from build123d import *

# Parameters (mm, degrees)
SKETCH1_W                                          = 14.224
SKETCH1_H                                          = 8.636
CBORE_FOR_M2_5_HEX_HEAD_MACHINE_SCREW1_D           = 3.048
CBORE_FOR_M2_5_HEX_HEAD_MACHINE_SCREW1_CBORE_D     = 4.7752
CBORE_FOR_M2_5_HEX_HEAD_MACHINE_SCREW1_CBORE_DEPTH = 3.048
M2_5_CLEARANCE_HOLE1_D                             = 3.048
M2_5_CLEARANCE_HOLE1_DEPTH                         = 2.54
M13_CLEARANCE_HOLE1_D                              = 15.494
M13_CLEARANCE_HOLE1_DEPTH                          = 2.54
CBORE_FOR_M3_5_HEX_HEAD_MACHINE_SCREW1_D           = 3.96748
CBORE_FOR_M3_5_HEX_HEAD_MACHINE_SCREW1_DEPTH       = 7.112
CBORE_FOR_M3_5_HEX_HEAD_MACHINE_SCREW1_CBORE_D     = 7.9375
CBORE_FOR_M3_5_HEX_HEAD_MACHINE_SCREW1_CBORE_DEPTH = 0.508
CBORE_FOR_M3_5_HEX_HEAD_MACHINE_SCREW1_TIP         = 1.145312823
CHAMFER1_SIZE                                      = 0.42926


with BuildPart() as part:
    # Sketch1 → Revolve1 (revolve)
    with BuildSketch(Plane(origin=(0, 0, 0), x_dir=(-1, 0, 0), z_dir=(0, 0, -1)), mode=Mode.PRIVATE) as revolve1_sk:
        with Locations((-7.112, 4.318)):
            Rectangle(SKETCH1_W, SKETCH1_H)
    revolve(revolve1_sk.sketch.rotate(Axis((0, 0, 0), (0, 1, 0)), 270), axis=Axis((0, 0, 0), (0, 1, 0)))

    # CBORE for M2.5 Hex Head Machine Screw1 (through all)
    with Locations(Plane(origin=(0, 8.636, 0), x_dir=(1, 0, 0), z_dir=(0, 1, 0))):
        with Locations((0, -11.176), (0, 11.176)):
            CounterBoreHole(CBORE_FOR_M2_5_HEX_HEAD_MACHINE_SCREW1_D / 2, CBORE_FOR_M2_5_HEX_HEAD_MACHINE_SCREW1_CBORE_D / 2, CBORE_FOR_M2_5_HEX_HEAD_MACHINE_SCREW1_CBORE_DEPTH)

    # M2.5 Clearance Hole1
    with Locations(Plane(origin=(0, 0, 0), x_dir=(-1, 0, 0), z_dir=(0, -1, 0))):
        with Locations((-7.902625387, 7.902625387), (7.902625387, -7.902625387), (-7.902625387, -7.902625387), (7.902625387, 7.902625387)):
            Hole(M2_5_CLEARANCE_HOLE1_D / 2, depth=M2_5_CLEARANCE_HOLE1_DEPTH)

    # M13 Clearance Hole1
    with Locations(Plane(origin=(0, 0, 0), x_dir=(-1, 0, 0), z_dir=(0, -1, 0))):
        with Locations((0, 0)):
            Hole(M13_CLEARANCE_HOLE1_D / 2, depth=M13_CLEARANCE_HOLE1_DEPTH)

    # CBORE for M3.5 Hex Head Machine Screw1
    with Locations(Plane(origin=(-14.224, 5.08, 0), x_dir=(0, 0, -1), z_dir=(-1, 0, 0))):
        with Locations((0, 0)):
            CounterBoreHole(CBORE_FOR_M3_5_HEX_HEAD_MACHINE_SCREW1_D / 2, CBORE_FOR_M3_5_HEX_HEAD_MACHINE_SCREW1_CBORE_D / 2, CBORE_FOR_M3_5_HEX_HEAD_MACHINE_SCREW1_CBORE_DEPTH, depth=CBORE_FOR_M3_5_HEX_HEAD_MACHINE_SCREW1_DEPTH)
            with Locations((0, 0, -(CBORE_FOR_M3_5_HEX_HEAD_MACHINE_SCREW1_DEPTH + CBORE_FOR_M3_5_HEX_HEAD_MACHINE_SCREW1_TIP / 2))):  # 120° drill point
                Cone(0, CBORE_FOR_M3_5_HEX_HEAD_MACHINE_SCREW1_D / 2, CBORE_FOR_M3_5_HEX_HEAD_MACHINE_SCREW1_TIP, mode=Mode.SUBTRACT)

    # Chamfer1
    chamfer1_edges = [part.edges().sort_by_distance(p)[0] for p in [
        (-13.716, 5.08, -1.98374),
    ]]
    chamfer(chamfer1_edges, length=CHAMFER1_SIZE)


solid = part.part
Can you work these out from the model? Positions are in its coordinate system, mm. A direction names the side the tool comes from. Coordinates: 2 decimals unless noted, no trailing zeros. Loops run counter-clockwise (first coordinate to the right, second up) from the corner with the lowest first, then second, coordinate; pieces in that order, holes last. Notation, with made-up numbers: M 66,51 L 115,51 A35 ccw 115,90 Z; hole C 42,-10 d11. An arc over 180 degrees is marked long. Return JSON: item names as keys, results as strings. Group by question number.
Item 1: Imagine slicing it at B-B (x = 0). Please give me the cut outline in (y, z), and give its area (3 significant figures).
Item 2: Imagine slicing it at A-A (z = 10). Please give me the cut outline in (x, y), and give its area (3 significant figures).
Item 3: Thinking about a two-plate mould opening in Z: for faces 1 (the flat face through (0, 8.636, 0)), 2 (the flat face through (-8, 2.54, 8)), which applies, released by +Z, released by -Z, zero draft, split by the parting line, or undercut?
Item 4: Imagine slicing it at C-C (x = -9). Please give me the cut outline in (y, z), and give its area (3 significant figures).
Item 5: I'm going to push flat-ended pins straight in: pin 1 Ø1.5 at (y, z) = (1.5, -1.5) entering from -X; pin 2 Ø1.8 at (x, z) = (7.9, 7.9) entering from -Y; pin 3 Ø4 at (x, z) = (0, 11.176) entering from -Y; pin 4 Ø4 at (y, z) = (4, 2) entering from -X. Where does each tip first touch, or does it pass through?
Item 6: Imagine slicing it at D-D (z = -4.25). Please give me the cut outline in (x, y).
Item 7: On a 3-axis mill with a long thin cutter (end or side, diameter ignored), from which of +Z, -Z, +X, -X, +Y, -Y can I reach the whole of each face in a straight line? I mean faces 3 (the flat face through (-8, 2.54, -8)), 4 (the flat face through (2, 5.588, -11)), 5 (the flat face through (-13.716, 3, -2)). Say none if no direction works.
Item 8: If I drill on L1, parallel to Z at x = 0, y = 6.9; L2, parallel to Y at x = -9.5, z = 0; L3, parallel to Z at x = 0, y = 1.65, over which ranges is the centre line in solid material (lowest first)? Write a range as from..to.
Verdict:
{
 "1": {"outline": "M 0,-14.22 L 8.64,-14.22 L 8.64,-13.56 L 5.59,-13.56 L 5.59,-12.7 L 0,-12.7 Z; M 0,-9.65 L 5.59,-9.65 L 5.59,-8.79 L 8.64,-8.79 L 8.64,8.79 L 5.59,8.79 L 5.59,9.65 L 0,9.65 L 0,7.75 L 2.54,7.75 L 2.54,-7.75 L 0,-7.75 Z; M 0,12.7 L 5.59,12.7 L 5.59,13.56 L 8.64,13.56 L 8.64,14.22 L 0,14.22 Z", "area": "143 mm^2"},
 "2": {"outline": "M -10.12,0 L -0.97,0 L -0.97,5.59 L -2.08,5.59 L -2.08,8.64 L -10.12,8.64 Z; M 0.97,0 L 10.12,0 L 10.12,8.64 L 2.08,8.64 L 2.08,5.59 L 0.97,5.59 Z", "area": "151 mm^2"},
 "3": {"face 1": "zero draft", "face 2": "undercut"},
 "4": {"outline": "M 0,-11.01 L 8.64,-11.01 L 8.64,11.01 L 0,11.01 L 0,8.96 L 2.54,8.96 L 2.54,6.85 L 0,6.85 L 0,-6.85 L 2.54,-6.85 L 2.54,-8.96 L 0,-8.96 Z; hole C 5.08,0 d3.97", "area": "167 mm^2"},
 "5": {"pin 1": "stops at x = -14.2", "pin 2": "stops at y = 2.54", "pin 3": "stops at y = 0", "pin 4": "stops at x = -13.98"},
 "6": {"outline": "M -13.57,0 L -6.48,0 L -6.48,2.54 L 6.48,2.54 L 6.48,0 L 13.57,0 L 13.57,8.64 L -13.57,8.64 Z"},
 "7": {"face 3": "-Y", "face 4": "+Y", "face 5": "-X"},
 "8": {"L1": "z = -14.22..-13.56, -8.79..8.79, 13.56..14.22", "L2": "y = 0..3.1, 7.06..8.64", "L3": "z = -14.22..-12.7, -9.65..-7.75, 7.75..9.65, 12.7..14.22"}
}
